Build history of the part. All positions in model axes, mm. A direction names the side the tool comes from. Round coordinates to 2 decimals unless told otherwise and drop trailing zeros. Write each loop counter-clockwise with the first axis right and the second up, starting at its lowest first coordinate (ties: lowest second). Pieces come first, ordered by that corner, then holes.
1) Saw through at D-D (x = 9). Write the cut outline in (y, z).
2) Wall check: probe 1 along Y at (x, z) = (0, 3.7) (3 decimals); probe 2 along X at (y, z) = (6, 2.8); probe 3 along Y at (x, z) = (0, 0.2) (3 decimals). Give the ranges that are in metal, low to high.
3) Saw through at A-A (y = 5). Write the cut outline in (x, z).
4) Pull direction X, two halves, no side cores. Call faces 1 (the cylindrical face through (-12.88, 11.81, 2.46)), 2 (the cylindrical face through (-0.202, -12.463, 4.028)), 3 (the flat face through (8, 0, 0)): +X half, -X half, draft (parallel to the pull), parting line (faces both ways), or undercut.
5) Which spindle directions (+Z, -Z, +X, -X, +Y, -Y) get a long thin tool onto all of the face, cutting with end or side? Do faces 4 (the cylindrical face through (6.466, -2.681, 0.246)), 5 (the cylindrical face through (-10.69, 6.41, 4.03)), 6 (the flat face through (-11, -14, 5)). Say none if no direction does.
6) Flat gauge pins, fed straight in: pin 1 (17.5 mm diameter, centred on x = -1, y = 1, fed in from +Z); pin 2 (0.9 mm diameter, centred on x = 12, y = 6.5, fed in from +Z); pin 3 (1 mm diameter, centred on y = 7.5, z = 1.5, fed in from +X); pin 4 (9.5 mm diameter, centred on x = 0, y = 0, fed in from +Z). Where does each tip first touch, or does it go through?
7) Saw through at B-B (x = 4). Write the cut outline in (y, z).
8) Saw through at C-C (y = -11.5). Write the cut outline in (x, z).
from build123d import *

# Parameters (mm, degrees)
SKETCH1_R           = 17.475
SKETCH1_R_2         = 8.025
BOSS_EXTRUDE1_DEPTH = 6
CUT_EXTRUDE1_START  = 6
SKETCH1_3_R         = 1.55
CUT_EXTRUDE1_DEPTH  = 4
BOSS_EXTRUDE2_START = 6
SKETCH2_R           = 18.5
SKETCH2_R_2         = 17.25
BOSS_EXTRUDE2_DEPTH = 1
SKETCH2_3_R         = 8.25
SKETCH2_3_R_2       = 7
BOSS_EXTRUDE3_DEPTH = 0.5


with BuildPart() as part:
    # Sketch1 → Boss-Extrude1 (new body)
    with BuildSketch(Plane.XY):
        Circle(SKETCH1_R)
        Circle(SKETCH1_R_2, mode=Mode.SUBTRACT)
    extrude(amount=BOSS_EXTRUDE1_DEPTH)

    # Sketch1<3> → Cut-Extrude1 (cut)
    with BuildSketch(Plane.XY.offset(CUT_EXTRUDE1_START)):
        with Locations((-12.124355653, 7)):
            Circle(SKETCH1_3_R)
        with BuildLine():
            ThreePointArc((0, 15.55), (-1.55, 14), (0, 12.45))
            Line((0, 12.45), (0, 15.55))
        make_face()
        with BuildLine():
            Line((0, 15.55), (0, 12.45))
            ThreePointArc((0, 12.45), (1.096015511, 12.903984489), (1.55, 14))
            ThreePointArc((1.55, 14), (1.096015511, 15.096015511), (0, 15.55))
        make_face()
        with Locations((12.124355653, 7)):
            Circle(SKETCH1_3_R)
        with Locations((12.124355653, -7)):
            Circle(SKETCH1_3_R)
        with Locations((0, -14)):
            Circle(SKETCH1_3_R)
        with Locations((-12.124355653, -7)):
            Circle(SKETCH1_3_R)
    extrude(amount=-CUT_EXTRUDE1_DEPTH, mode=Mode.SUBTRACT)

    # Sketch2 → Boss-Extrude2 (add)
    with BuildSketch(Plane.XY.offset(BOSS_EXTRUDE2_START)):
        Circle(SKETCH2_R)
        Circle(SKETCH2_R_2, mode=Mode.SUBTRACT)
    extrude(amount=-BOSS_EXTRUDE2_DEPTH)

    # Sketch2<3> → Boss-Extrude3 (add)
    with BuildSketch(Plane.XY):
        Circle(SKETCH2_3_R)
        Circle(SKETCH2_3_R_2, mode=Mode.SUBTRACT)
    extrude(amount=BOSS_EXTRUDE3_DEPTH)


solid = part.part
Evaluation:
1. outline: (-16.16, 5) - (-14.98, 5) - (-14.98, 0) - (14.98, 0) - (14.98, 5) - (16.16, 5) - (16.16, 6) - (-16.16, 6) - close
2. probe 1: y = -17.475 to -15.55, -12.45 to -8.025, 8.025 to 12.45, 15.55 to 17.475
2. probe 2: x = -16.41 to -13.31, -10.94 to -5.33, 5.33 to 10.94, 13.31 to 16.41
2. probe 3: y = -17.475 to -7, 7 to 17.475
3. outline: (-17.81, 5) - (-16.74, 5) - (-16.74, 0) - (-4.9, 0) - (-4.9, 0.5) - (-6.28, 0.5) - (-6.28, 6) - (-17.81, 6) - close; (4.9, 0) - (16.74, 0) - (16.74, 5) - (17.81, 5) - (17.81, 6) - (6.28, 6) - (6.28, 0.5) - (4.9, 0.5) - close
4. face 1: parting line
4. face 2: undercut
4. face 3: draft
5. face 4: +Z, -Z
5. face 5: +Z
5. face 6: -Z
6. pin 1: stops at z = 6
6. pin 2: stops at z = 2
6. pin 3: stops at x = 16.01
6. pin 4: passes through
7. outline: (-18.06, 5) - (-17.01, 5) - (-17.01, 0) - (-5.74, 0) - (-5.74, 0.5) - (-6.96, 0.5) - (-6.96, 6) - (-18.06, 6) - close; (5.74, 0) - (17.01, 0) - (17.01, 5) - (18.06, 5) - (18.06, 6) - (6.96, 6) - (6.96, 0.5) - (5.74, 0.5) - close
8. outline: (-14.49, 5) - (-13.16, 5) - (-13.16, 0) - (13.16, 0) - (13.16, 5) - (14.49, 5) - (14.49, 6) - (-14.49, 6) - close
